Input: part model. Units: mm. Frame: model coordinates. Face numbers are marked on the shaded views. Coordinates: 2 decimals unless noted, no trailing zeros. Loops run counter-clockwise (first coordinate to the right, second up) from the corner with the lowest first, then second, coordinate; pieces in that order, holes last. Notation, with made-up numbers: (44.5, 27.5) - (54.5, 27.5) arc R20 ccw to (54.5, 58.5) - close; hole circle Ø7 at (-15.5, 29). An arc over 180 degrees is marked (long way). Use a Markdown table: item, result. Add a question column.
1. Ray query, L1, parallel to Y at x = -2, z = 14; L2, parallel to Z at x = 0.25, y = 20.5; L3, parallel to Z at x = 3.25, y = 25. Return the intervals inside material, ascending. Write a range as [from, to].
2. Section query C-C on z = -2. Return the cut outline in (x, y).
3. Section query B-B on x = -2. Return the cut outline in (y, z), then the cut area to 3 significant figures.
4. Section query D-D on z = -16.5. Return the cut outline in (x, y), then the cut area to 3 significant figures.
5. Contact query for flat-ended pins moving along their axis: P1, Ø1.6, axis at x = 2, y = 1, coming from the +Z side; P2, Ø0.6, axis at x = -1, y = 1.5, coming from the -Z side; P3, Ø1, axis at y = 1, z = 3.5, coming from the -X side. Output: stop coordinate, or through.
6. Draft query along Z for the marked faces 1, 2 and 3. Return one class per face: released by +Z, released by -Z, zero draft, split by the parting line, or undercut.
Autodesk Inventor part; units mm, degrees
ref_plane "YZ Plane" through (0, 0, 0) normal (1, 0, 0) x (0, 1, 0)
ref_plane "XZ Plane" through (0, 0, 0) normal (0, 1, 0) x (-1, 0, 0)
ref_plane "XY Plane" through (0, 0, 0) normal (0, 0, 1) x (1, 0, 0)
sketch "Sketch1" plane through (0, 0, 0) normal (0, 1, 0) x (-1, 0, 0)
  line L0 (3, 12) -> (-4, 12)
  line L1 (-4, 12) -> (-4, -10.3)
  line L2 (-4, -10.3) -> (3, -10.3)
  line L3 (3, -10.3) -> (3, 12)
  point P0 (0, 0)
  dimension "d0" = 7
  dimension "d1" = 22.3
extrude "Extrusion1" add sketch "Sketch1" along normal blind 2
sketch "Sketch2" plane through (0, 2, 0) normal (0, 1, 0) x (1, 0, 0)
  line L0 (-5, -24) -> (4, -24)
  line L1 (4, -24) -> (4, 21.5)
  line L2 (4, 21.5) -> (-5, 21.5)
  line L3 (-5, 21.5) -> (-5, -24)
  point P0 (0, 0)
  dimension "d4" = 45.5
extrude "Extrusion2" add sketch "Sketch2" along normal blind 30
sketch "Sketch3" plane through (4, 0, 12) normal (1, 0, 0) x (0, 0, -1)
  circle A0 centre (-2, 22) radius 8
  circle A1 centre (24, 22) radius 8
  point P0 (12, 0)
  dimension "d7" = 16
  dimension "d8" = 16
  dimension "d9" = 10
extrude "Extrusion3" cut sketch "Sketch3" against normal blind 30
fillet "Fillet1" radius 2 10 edges at (-0.5, 32, 24) (4, 32, 1.25) (-0.5, 32, -21.5) (-5, 32, 1.25) (-0.5, 2, 24) (4, 17, 24) (-5, 17, 24) (-0.5, 2, -21.5) (-5, 17, -21.5) (4, 17, -21.5)
properties part number "sonarMount"
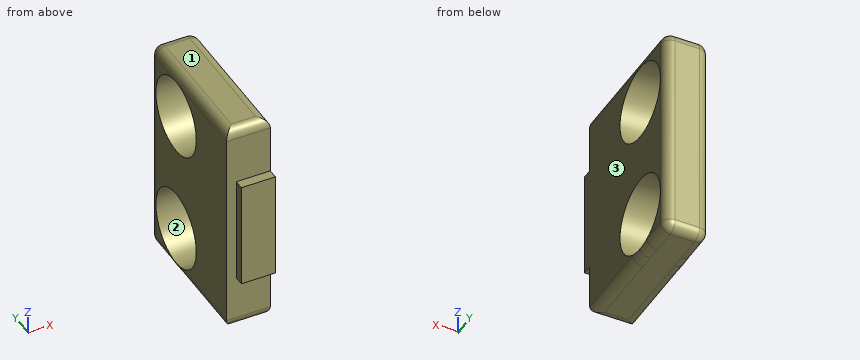
Resolved:
| question | item | result |
|---|---|---|
| 1 | L1 | [2, 14], [30, 32] |
| 1 | L2 | [-21.5, -19.86], [-4.14, 6.14], [21.86, 24] |
| 1 | L3 | [-21.06, -19.42], [-4.58, 6.58], [21.42, 23.56] |
| 2 | outline | (-5, 2) - (-3, 2) - (-3, 0) - (4, 0) - (4, 30) arc R2 ccw to (2, 32) - (-3, 32) arc R2 ccw to (-5, 30) - close |
| 3 | outline | (0, -10.3) - (2, -10.3) - (2, -19.5) arc R2 ccw to (4, -21.5) - (30, -21.5) arc R2 ccw to (32, -19.5) - (32, 22) arc R2 ccw to (30, 24) - (4, 24) arc R2 ccw to (2, 22) - (2, 12) - (0, 12) - close; hole circle Ø16 at (22, -12); hole circle Ø16 at (22, 14) |
| 3 | area | 1,000 mm² |
| 4 | outline | (-5, 2) - (4, 2) - (4, 15.39) - (-5, 15.39) - close; (-5, 28.61) - (4, 28.61) - (4, 30) arc R2 ccw to (2, 32) - (-3, 32) arc R2 ccw to (-5, 30) - close |
| 4 | area | 149 mm² |
| 5 | P1 | z = 12 |
| 5 | P2 | z = -10.3 |
| 5 | P3 | x = -3 |
| 6 | face 1 | released by +Z |
| 6 | face 2 | undercut |
| 6 | face 3 | zero draft |
